```python
from build123d import *

# Parameters (mm, degrees)
F0_R     = 2.5
F1_DEPTH = 15
F3_DEPTH = 10


with BuildPart() as f1:
    # F0 (on Top) → F1 (new body)
    with BuildSketch(Plane.XY):
        with BuildLine():
            ThreePointArc((-17.907068, 5), (-20.407068, 7.5), (-22.907068, 5))
            ThreePointArc((-22.907068, 5), (-20.407068, 2.5), (-17.907068, 5))
        make_face()
        with Locations((14.592932, 5)):
            Circle(F0_R)
        Polygon((22.092932, 10), (-27.907068, 10), (-27.907068, 5), (-27.907068, 0), (22.092932, 0), (22.092932, 5), align=None)
        with BuildLine():
            ThreePointArc((-17.907068, 5), (-20.407068, 2.5), (-22.907068, 5))
            ThreePointArc((-22.907068, 5), (-20.407068, 7.5), (-17.907068, 5))
        make_face(mode=Mode.SUBTRACT)
        with Locations((14.592932, 5)):
            Circle(F0_R, mode=Mode.SUBTRACT)
    extrude(amount=F1_DEPTH)

    # F2 (on Front) → F3 (cut)
    with BuildSketch(Plane.XZ):
        with BuildLine():
            Line((7.092932, 15), (-12.907068, 15))
            ThreePointArc((-12.907068, 15), (-2.907068, 5), (7.092932, 15))
        make_face()
    extrude(amount=-F3_DEPTH, mode=Mode.SUBTRACT)


solid = f1.part
```
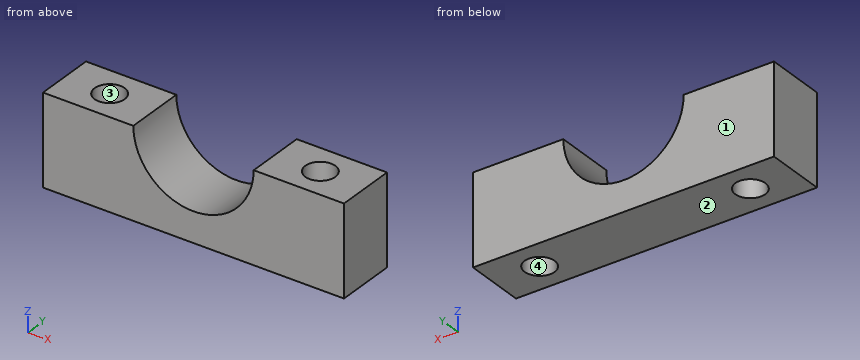
Work out the finished part from the listing and answer in its coordinate system (mm). Face numbers are marked on the shaded views. Coordinates: 2 decimals unless noted, no trailing zeros. Order: outer loops, then holes, each group sorted by start corner. A loop starts at its lowest first (then second) coordinate and runs counter-clockwise, first axis right, second up. Notation, with made-up numbers: M -27,30.5 L -6,30.5 A24 ccw -6,48.5 Z; hole C 63.25,50 d7. An arc over 180 degrees is marked long. Use CSV: the item, a comma, the result in double quotes.
1) Section D-D on z = 3 is taken. Write down the section's boundary in (x, y).
Worked out:
outline,"M -27.91,0 L 22.09,0 L 22.09,10 L -27.91,10 Z; hole C -20.41,5 d5; hole C 14.59,5 d5"
2) Section A-A on z = 7 is taken. Write down the section's boundary in (x, y), plus the area to 3 significant figures.
Worked out:
outline,"M -27.91,0 L -8.91,0 L -8.91,10 L -27.91,10 Z; M 3.09,0 L 22.09,0 L 22.09,10 L 3.09,10 Z; hole C -20.41,5 d5; hole C 14.59,5 d5"
area,"341 mm^2"
3) Determine the mould class of the marked faces 1, 2, 3 and 4 for opening direction Y: released by +Y, released by -Y, zero draft, split by the parting line, or undercut.
Worked out:
face 1,"released by +Y"
face 2,"zero draft"
face 3,"undercut"
face 4,"undercut"
4) Section B-B on y = 5 is taken. Write down the section's boundary in (x, z), plus the area to 3 significant figures.
Worked out:
outline,"M -27.91,0 L -22.91,0 L -22.91,15 L -27.91,15 Z; M -17.91,0 L 12.09,0 L 12.09,15 L 7.09,15 A10 cw -12.91,15 L -17.91,15 Z; M 17.09,0 L 22.09,0 L 22.09,15 L 17.09,15 Z"
area,"443 mm^2"
5) Section C-C on y = 1 is taken. Write down the section's boundary in (x, z), plus the area to 3 significant figures.
Worked out:
outline,"M -27.91,0 L 22.09,0 L 22.09,15 L 7.09,15 A10 cw -12.91,15 L -27.91,15 Z"
area,"593 mm^2"
6) Consider line 1 (X direction, y = 2.75, z = 10); line 2 (X direction, y = 3.5, z = 12.75); line 3 (X direction, y = 5.25, z = 1.25). Determine where each line is inside the solid, lowest interval first. Write a range as [from, to].
Worked out:
line 1,"x = [-27.91, -21.5], [-19.32, -11.57], [5.75, 13.5], [15.68, 22.09]"
line 2,"x = [-27.91, -22.41], [-18.41, -12.65], [6.84, 12.59], [16.59, 22.09]"
line 3,"x = [-27.91, -22.89], [-17.92, 12.11], [17.08, 22.09]"
